Part model, mm, in its own coordinate system. Face numbers are marked on the shaded views. A direction names the side the tool comes from. Round coordinates to 2 decimals unless told otherwise and drop trailing zeros. Write each loop counter-clockwise with the first axis right and the second up, starting at its lowest first coordinate (ties: lowest second). Pieces come first, ordered by that corner, then holes. Notation, with made-up numbers: M 30.25,88.5 L 85.25,88.5 A4 ccw 85.25,94.5 Z; hole C -30,-1 d8. An arc over 180 degrees is marked long. Use one line per item in the form item = value. Start each with the question number.
Item 1: Cut at C-C, the plane x = 128. Give the cut face in (y, z), then the cut area to 3 significant figures.
Item 2: Cut at A-A, the plane z = 30. Give the cut face in (x, y).
Item 3: Probe L1, parallel to Z at x = 40.15, y = 17.5; L2, parallel to X at y = -22, z = 49.5; L3, parallel to X at y = -22, z = 6. List the from-to ranges inside material, lowest first.
Item 4: Cut at B-B, the plane z = 45. Give the cut face in (x, y), then the cut area to 3 significant figures.
Item 5: Which spindle directions (+Z, -Z, +X, -X, +Y, -Y) get a long thin tool onto all of the face, cutting with end or side? Do the marked faces 1, 2 and 3. Say none if no direction does.
Item 6: Mould opens along X. For the marked faces 4, 5 and 6 say: +X half, -X half, draft (parallel to the pull), parting line (faces both ways), or undercut.
Item 7: Flat gauge pins, fed straight in: pin 1 Ø1 at (x, y) = (94, -25.5) entering from -Z; pin 2 Ø3.5 at (x, z) = (42.5, 34) entering from -Y; pin 3 Ø1.5 at (x, z) = (42, 26.5) entering from +Y; pin 4 Ø8 at (y, z) = (-12.5, 15) entering from +X. Where does each tip first touch, or does it go through?
Item 8: Cut at D-D, the plane y = 17.5. State how many separate pieces and enclosed holes the cut face has, then the cut area to 3 significant figures.
from build123d import *

# Parameters (mm, degrees)
CYLINDER035_R          = 12.5
CYLINDER035_DEPTH      = 25
CYLINDER034_R          = 2.5
CYLINDER034_DEPTH      = 8
BOX022_W               = 45
BOX022_H               = 50
BOX022_DEPTH           = 2.5
CUT042_ROLL_ANGLE      = 90
CUT042_PLACEMENT_ANGLE = 90
BOX013_W               = 35
BOX013_H               = 56
BOX013_DEPTH           = 4
BOX002_W               = 162
BOX002_H               = 70
BOX002_DEPTH           = 5
CHAMFER_SIZE           = 4
CHAMFER001_SIZE        = 4


with BuildPart() as hueco_rotor001:
    # Cylinder035 → Cylinder035 (new body)
    with BuildSketch(Plane(origin=(25, 2.5, 30), x_dir=(0, 0, -1), z_dir=(1, 0, 0))):
        Circle(CYLINDER035_R)
    extrude(amount=CYLINDER035_DEPTH)


with BuildPart() as obj1:
    # Cylinder034 → Cylinder034 (new body)
    with BuildSketch(Plane(origin=(10, 10, 38), x_dir=(1, 0, 0), z_dir=(0, 0, 1))):
        Circle(CYLINDER034_R)
    extrude(amount=CYLINDER034_DEPTH)


with BuildPart() as obj2:
    # Link025 base: copy of obj1
    add(obj1.part)


with BuildPart() as obj2_1:
    # Link025 placement: moved
    add(obj2.part.moved(Location((0, 30, 0))))


with BuildPart() as obj3:
    # Link024 base: copy of obj1
    add(obj1.part)


with BuildPart() as obj3_1:
    # Link024 placement: moved
    add(obj3.part.moved(Location((30, 0, 0))))


with BuildPart() as obj4:
    # Link023 base: copy of obj1
    add(obj1.part)


with BuildPart() as obj4_1:
    # Link023 placement: moved
    add(obj4.part.moved(Location((30, 30, 0))))


with BuildPart() as union_base_motor:
    # Box022 → Box022 (new body)
    with BuildSketch(Plane.XY.offset(40)):
        with Locations((22.5, 25)):
            Rectangle(BOX022_W, BOX022_H)
    extrude(amount=BOX022_DEPTH)

    # Cut039: cut obj4
    add(obj4_1.part, mode=Mode.SUBTRACT)

    # Cut040: cut obj3
    add(obj3_1.part, mode=Mode.SUBTRACT)

    # Cut041: cut obj2
    add(obj2_1.part, mode=Mode.SUBTRACT)

    # Cut042: cut obj1
    add(obj1.part, mode=Mode.SUBTRACT)


with BuildPart() as union_base_motor_1:
    # Cut042 roll: moved
    add(union_base_motor.part.rotate(Axis((0, 0, 0), (1, 0, 0)), CUT042_ROLL_ANGLE))


with BuildPart() as union_base_motor_2:
    # Cut042 placement: moved
    add(union_base_motor_1.part.moved(Location((0, -22.5, 5))).rotate(Axis((0, -22.5, 5), (0, 0, 1)), CUT042_PLACEMENT_ANGLE))

    # Cut043: cut Hueco rotor001
    add(hueco_rotor001.part, mode=Mode.SUBTRACT)


with BuildPart() as union_base_motor_3:
    # Cut043 placement: moved
    add(union_base_motor_2.part.moved(Location((-1, 0, 0))))


with BuildPart() as soporte_motor:
    # Box013 → Box013 (new body)
    with BuildSketch(Plane(origin=(0, -28, 5), x_dir=(1, 0, 0), z_dir=(0, 0, 1))):
        with Locations((17.5, 28)):
            Rectangle(BOX013_W, BOX013_H)
    extrude(amount=BOX013_DEPTH)


with BuildPart() as obj5:
    # Box002 → Box002 (new body)
    with BuildSketch(Plane(origin=(0, -35, 0), x_dir=(1, 0, 0), z_dir=(0, 0, 1))):
        with Locations((81, 35)):
            Rectangle(BOX002_W, BOX002_H)
    extrude(amount=BOX002_DEPTH)


with BuildPart() as base:
    # Link011 base: copy of soporte motor
    add(soporte_motor.part)


with BuildPart() as base_1:
    # Link011 placement: moved
    add(base.part.moved(Location((127.000053, -2e-06, -2e-06))))

    # Fusion008: union soporte motor, obj5
    add(soporte_motor.part)
    add(obj5.part)


with BuildPart() as base_2:
    # Fusion008 placement: moved
    add(base_1.part.moved(Location((-7, 0, 0))))


with BuildPart() as chamfer001:
    # Link base: copy of union base motor
    add(union_base_motor_3.part)


with BuildPart() as chamfer001_1:
    # Link placement: moved
    add(chamfer001.part.moved(Location((67.5, -8e-06, 0))))

    # Fusion063: union union base motor, Base
    add(union_base_motor_3.part)
    add(base_2.part)

    # Chamfer
    chamfer_edges = [chamfer001_1.edges().sort_by_distance(p)[0] for p in [
        (41.5, 0, 5),
    ]]
    chamfer(chamfer_edges, length=CHAMFER_SIZE)

    # Chamfer001
    chamfer001_edges = [chamfer001_1.edges().sort_by_distance(p)[0] for p in [
        (106.5, -8e-06, 5),
    ]]
    chamfer(chamfer001_edges, length=CHAMFER001_SIZE)


solid = chamfer001_1.part
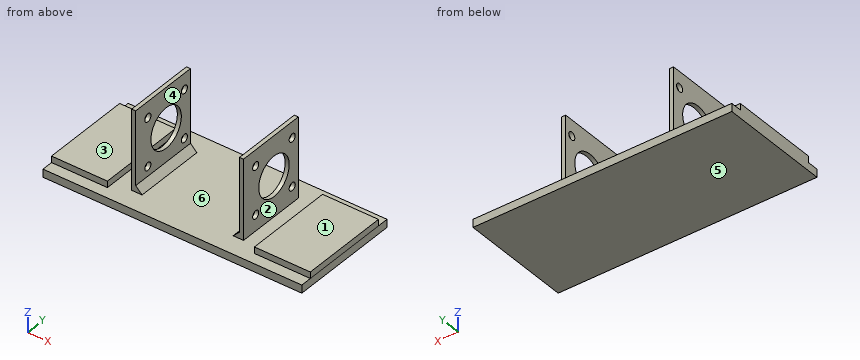
Model answer:
q1.outline = M -35,0 L 35,0 L 35,5 L 28,5 L 28,9 L -28,9 L -28,5 L -35,5 Z
q1.area = 574 mm²
q2.outline = M 39,-22.5 L 41.5,-22.5 L 41.5,-10 L 39,-10 Z; M 39,15 L 41.5,15 L 41.5,22.5 L 39,22.5 Z; M 106.5,-22.5 L 109,-22.5 L 109,-10 L 106.5,-10 Z; M 106.5,15 L 109,15 L 109,22.5 L 106.5,22.5 Z
q3.L1 = 0 to 12.5, 17.5 to 42.5, 47.5 to 55
q3.L2 = 39 to 41.5, 106.5 to 109
q3.L3 = -7 to 28, 39 to 44.5, 103.5 to 109, 120 to 155
q4.outline = M 39,-22.5 L 41.5,-22.5 L 41.5,-15 L 39,-15 Z; M 39,-10 L 41.5,-10 L 41.5,15 L 39,15 Z; M 39,20 L 41.5,20 L 41.5,22.5 L 39,22.5 Z; M 106.5,-22.5 L 109,-22.5 L 109,-15 L 106.5,-15 Z; M 106.5,-10 L 109,-10 L 109,15 L 106.5,15 Z; M 106.5,20 L 109,20 L 109,22.5 L 106.5,22.5 Z
q4.area = 175 mm²
q5.face_1 = +Z, +X, +Y, -Y
q5.face_2 = +Z, +Y, -Y
q5.face_3 = +Z, -X, +Y, -Y
q6.face_4 = undercut
q6.face_5 = draft
q6.face_6 = undercut
q7.pin_1 = 0
q7.pin_2 = -22.5
q7.pin_3 = 22.5
q7.pin_4 = 109
q8.separate_pieces = 5
q8.enclosed_holes = 0
q8.area = 1,310 mm²
